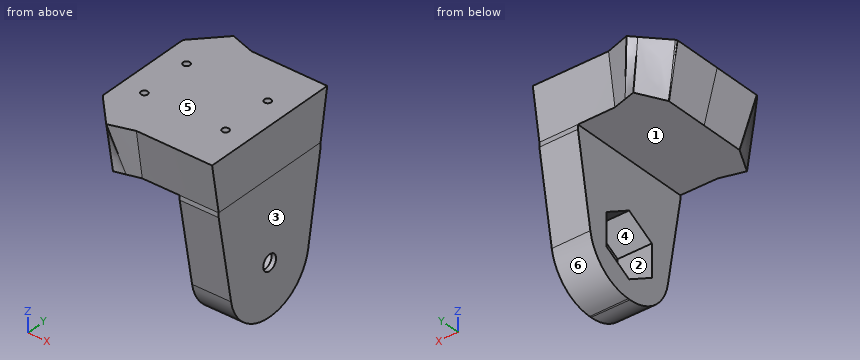
Autodesk Fusion 360 part; units mm, degrees
sketch "Support moteur/Cam" plane through (0, 0, 0) normal (0, 0, 1) x (1, 0, 0)
  line L0 (-113.5546, -207.3984) -> (-130.3546, -207.3984)
  line L1 (-130.3546, -207.3984) -> (-135.6849, -205.7263)
  line L2 (-135.6849, -205.7263) -> (-141.4789, -211.9329)
  line L3 (-141.4789, -211.9329) -> (-141.6802, -212.3176)
  line L4 (-141.6802, -212.3176) -> (-141.6802, -223.1)
  line L5 (-113.5528, -238.7984) -> (-130.3528, -238.8003)
  line L6 (-130.3528, -238.8003) -> (-135.6829, -240.4729)
  line L7 (-141.4776, -234.267) -> (-141.679, -233.8823)
  line L8 (-141.679, -233.8823) -> (-141.6802, -223.1)
  line L9 (-135.6829, -240.4729) -> (-141.4776, -234.267)
  circle A0 centre (-136.6035, -217.4087) radius 0.75
  circle A1 centre (-118.6035, -217.4087) radius 0.75
  circle A2 centre (-136.6035, -228.9087) radius 0.75
  circle A3 centre (-118.6035, -228.9087) radius 0.75
  line L10 (-113.5546, -207.3984) -> (-113.5528, -238.7984)
  line L11 (-141.6802, -223.1) -> (-113.5537, -223.0984)
  point P0 (-136.6035, -217.4087)
  point P1 (-118.6035, -217.4087)
  point P2 (-118.6035, -228.9087)
  point P3 (-136.6035, -228.9087)
  dimension "d217" = 16.8
  dimension "d227" = 1.5
  dimension "d228" = 1.5
  dimension "d229" = 1.5
  dimension "d230" = 1.5
ref_plane "WorkPlane9" through (0, 0, -10.8) normal (0, 0, 1) x (1, 0, 0)
sketch "Support moteur/Cam2" plane through (0, 0, -10.8) normal (0, 0, 1) x (1, 0, 0)
  line L0 (-113.5546, -236.9984) -> (-130.3974, -237.1164)
  line L1 (-130.3974, -237.1164) -> (-135.6833, -238.6066)
  line L2 (-135.6833, -238.6066) -> (-138.7984, -232.7391)
  line L3 (-138.7984, -223.0984) -> (-138.7984, -232.7391)
  line L4 (-138.7984, -223.0984) -> (-138.7984, -213.4577)
  line L5 (-135.6833, -207.5901) -> (-138.7984, -213.4577)
  line L6 (-130.3974, -209.0804) -> (-135.6833, -207.5901)
  line L7 (-113.5546, -209.1984) -> (-130.3974, -209.0804)
  line L8 (-122.1546, -237.0587) -> (-122.1546, -209.1381)
  line L9 (-113.5546, -209.1984) -> (-113.5546, -236.9984)
  line L10 (-138.7984, -223.0984) -> (-113.5546, -223.0984) construction
  dimension "d221" = 8.6
loft "Loft1" add profiles "Support moteur/Cam2", "Support moteur/Cam" section 1 section 2 contours L0 L1 L2 L3 L4 L10 L11 | L5 L6 L7 L8 L9 L10 L11 | A0 | A1
extrude "Support Moteur/Cam" cut sketch "Support moteur/Cam" against normal blind 8 contours A0 | A1 | A2 | A3
extrude "Extrude10" add sketch "Support moteur/Cam2" against normal blind 29 contours L0 L7 L8 L9
chamfer "Chamfer3" distance 4.9 distance2 28 2 edges at (-117.8546, -209.1683, -39.8) (-117.8546, -237.0285, -39.8) measured on face at (-119.2879, -218.4651, -39.8) measured on face at (-119.2879, -218.4651, -39.8)
fillet "Fillet1" radius 10.5 2 edges at (-117.8546, -232.1284, -39.8) (-117.8546, -214.0684, -39.8)
sketch "Support moteur/Cam3" plane through (-122.1546, 0, 0) normal (-1, 0, 0) x (0, -1, 0)
  ellipse E0 centre (222.8605, -29.3) end of major axis (212.3603, -29.3) minor radius 10.5 (212.5175, -31.11) -> (222.8605, -39.8) ccw
  line L0 (222.8605, -39.8) -> (223.3362, -39.8)
  ellipse E1 centre (223.3362, -29.3) end of major axis (233.8365, -29.3) minor radius 10.5 (223.3362, -39.8) -> (233.6793, -31.11) ccw
  line L1 (233.6793, -31.11) -> (237.0587, -11.8)
  line L2 (237.0587, -11.8) -> (237.0587, -10.8)
  line L3 (237.0587, -10.8) -> (209.1381, -10.8)
  line L4 (209.1381, -10.8) -> (209.1381, -11.8)
  line L5 (209.1381, -11.8) -> (212.5175, -31.11)
  line L6 (223.0984, -10.8) -> (223.0984, -28.5) construction
  line L7 (229.2984, -32.0796) -> (229.2984, -24.9204)
  line L8 (229.2984, -24.9204) -> (223.0984, -21.3409)
  line L9 (223.0984, -21.3409) -> (216.8984, -24.9204)
  line L10 (216.8984, -24.9204) -> (216.8984, -32.0796)
  line L11 (216.8984, -32.0796) -> (223.0984, -35.6591)
  line L12 (223.0984, -35.6591) -> (229.2984, -32.0796)
  circle A0 centre (223.0984, -28.5) radius 1.75
  line L13 (223.0984, -10.8) -> (223.0984, -33.8) construction
  circle A1 centre (223.0984, -33.8) radius 1.6 construction
  circle A2 centre (223.0984, -33.8) radius 3.1 construction
  line L14 (217.8116, -36.9) -> (223.0984, -36.9) construction
  line L15 (221.2654, -36.3) -> (224.9314, -36.3)
  circle A3 centre (223.0984, -33.8) radius 4.1 construction
  point P0 (223.0984, -28.5)
  dimension "d233" = 17.7
  dimension "d235" = 12.4
  dimension "d236" = 3.5
  dimension "d380" = 23
  dimension "d381" = 3.2
  dimension "d382" = 6.2
  dimension "d383" = 0.6
  dimension "d384" = 8.2
  dimension "d395" = 9
extrude "Extrude12" cut sketch "Support moteur/Cam3" against normal through all contours A0
extrude "Extrude13" cut sketch "Support moteur/Cam3" against normal blind 7.6 contours L7 L8 L9 L10 L11 L12
extrude "Extrude19" [suppressed]
fillet "Fillet2" [suppressed]
For this review, take the finished solid that the model builds, in its own axes (mm). Face numbers are marked on the shaded views. A direction names the side the tool comes from. Coordinates: 2 decimals unless noted, no trailing zeros. Order: outer loops, then holes, each group sorted by start corner. A loop starts at its lowest first (then second) coordinate and runs counter-clockwise, first axis right, second up. Notation, with made-up numbers: (71, 84.5) -> (129, 84.5) arc R14 ccw to (129, 89.5) -> close; hole circle Ø1 at (-27, 56). An arc over 180 degrees is marked (long way). Use CSV: the item, a comma, the result in double quotes. Start each with the question number.
Item 1: Insertion check: pin 1 (2.5 mm diameter, centred on x = -136.6, y = -217.41, fed in from +Z); pin 2 (2.5 mm diameter, centred on x = -118.6, y = -228.91, fed in from -Z); pin 3 (2 mm diameter, centred on x = -121.5, z = -26.5, fed in from -Y); pin 4 (6 mm diameter, centred on y = -231.5, z = -5.5, fed in from -X). Each pin has a flat end and moves straight along its axis. Give the tip position at first contact, or say it passes through.
Item 2: We need section B-B, the plane z = -28.5. Give the boundary of the cut face in (x, y).
Item 3: Wall thickness on probe 1 along Z at (x, y) = (-136.5, -232.5); probe 2 along X at (y, z) = (-228.5, -30.5); probe 3 along X at (y, z) = (-225, -36.5): over which ranges is each line inside the solid? List them lowest first.
Item 4: For the marked faces 1, 2 and 3, list the 3-axis set-ups (+Z, -Z, +X, -X, +Y, -Y) from which the entire face can be reached by the end or side of a thin tool; tool diameter is ignored.
Item 5: We need section D-D, the plane z = -5. Give the number of separate pieces and of enclosed holes in the cut face, then the cut area to 3 significant figures.
Item 6: We need section C-C, the plane z = -35. Give the boundary of the cut face in (x, y), then the cut area to 3 significant figures.
Item 7: We need section A-A, the plane z = -23. Give the boundary of the cut face in (x, y), then the cut area to 3 significant figures.
Item 8: Draft analysis for pull direction Y (two halves, no side actions). For the marked faces 4, 5 and 6, state which applies: pulls with the +Y half, pulls with the -Y half, needs draft (parallel to the pull), parting line crosses it, or undercut.
Derived:
1,pin 1,"stops at z = 0"
1,pin 2,"stops at z = -38.86"
1,pin 3,"stops at y = -234.66"
1,pin 4,"stops at x = -141.01"
2,outline,"(-122.15, -234.14) -> (-113.55, -234.08) -> (-113.55, -224.85) -> (-114.55, -224.85) -> (-114.55, -229.3) -> (-122.15, -229.3) -> close; (-122.15, -216.9) -> (-114.55, -216.9) -> (-114.55, -221.35) -> (-113.55, -221.35) -> (-113.55, -212.12) -> (-122.15, -212.06) -> close"
3,probe 1,"z = -10.8 to 0"
3,probe 2,"x = -114.55 to -113.55"
3,probe 3,"x = -122.15 to -113.55"
4,face 1,"-Z, -X, +Y, -Y"
4,face 2,"-X"
4,face 3,"+Z, -Z, +X, +Y, -Y"
5,separate pieces,"1"
5,enclosed holes,"4"
5,area,"786 mm^2"
6,outline,"(-122.15, -232.15) -> (-113.55, -232.09) -> (-113.55, -214.1) -> (-122.15, -214.04) -> (-122.15, -221.96) -> (-114.55, -221.96) -> (-114.55, -224.24) -> (-122.15, -224.24) -> close"
6,area,"138 mm^2"
7,outline,"(-122.15, -235.1) -> (-113.55, -235.04) -> (-113.55, -211.16) -> (-122.15, -211.1) -> (-122.15, -220.22) -> (-114.55, -220.22) -> (-114.55, -225.97) -> (-122.15, -225.97) -> close"
7,area,"162 mm^2"
8,face 4,"undercut"
8,face 5,"needs draft"
8,face 6,"pulls with the +Y half"
